Study the drawing (mm; zero at the part's minimum x, y, z) and answer. A direction names the side the tool comes from. Give positions to 0.01 mm unless a question says otherwise; leave off trailing zeros. Write each loop counter-clockwise with the first axis right and the second up, starting at its lowest first coordinate (ties: lowest second). Pieces come first, ordered by that corner, then holes. Notation, with made-up numbers: (11, 36) - (36, 36) arc R23 cw to (36, 52) - close; hole circle Ø7 at (-17, 50.5). An arc over 180 degrees is marked (long way). One line per item, written item: value. Start each with the question number.
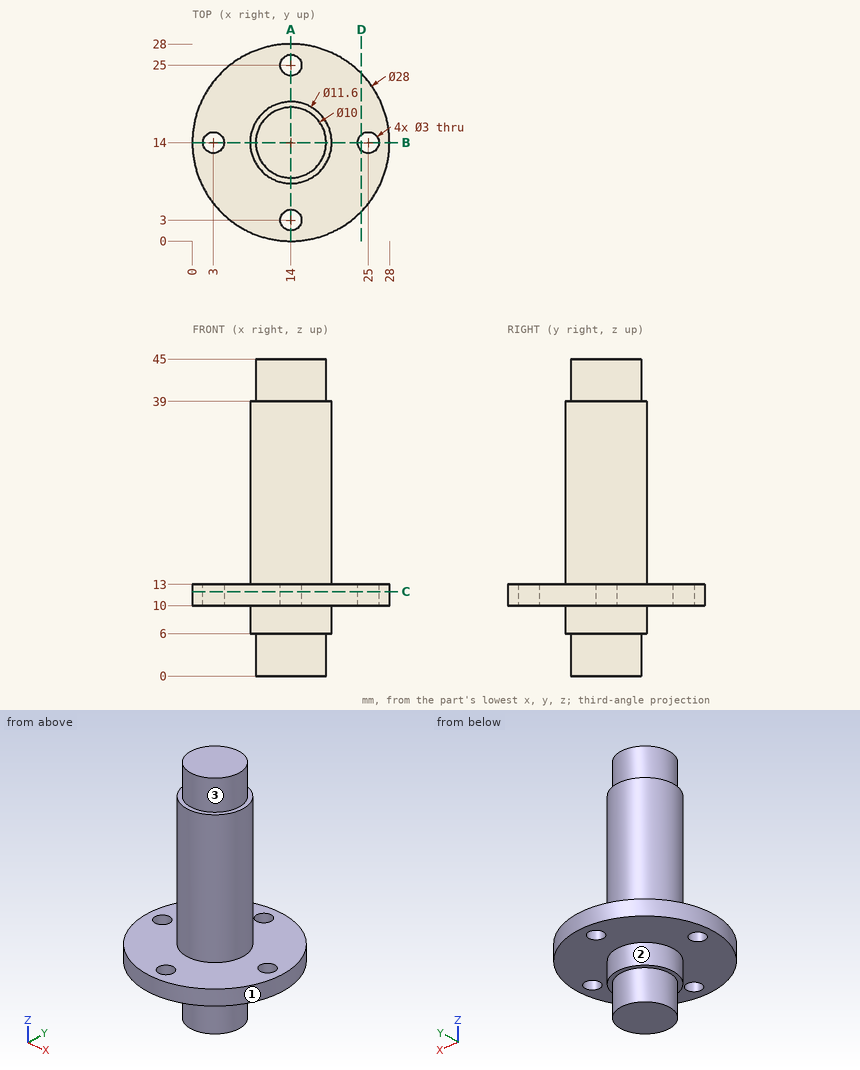
Item 1: For the marked faces 1, 2 and 3, determine the directions among +Z, -Z, +X, -X, +Y, -Y from which every point of the face is accessible in a straight line to the end or side of a thin tool.
Item 2: Each of these flat-tipped pins is pushed along its axis until it touches: pin 1 Ø10 at (y, z) = (23.5, 38) entering from +X; pin 2 Ø10 at (y, z) = (7.5, 7.5) entering from -X; pin 3 Ø5 at (x, y) = (3, 14) entering from +Z; pin 4 Ø13 at (x, y) = (13, 14.5) entering from -Z. Where does it stop, or does it pass through?
Item 3: Straight lines are drawn through the part: line 1 along Y through (x, z) = (14, 11.9); line 2 along Z through (x, y) = (16, 2); line 3 along Y through (x, z) = (3, 11.1). For each, find the intervals that lie inside material, in ascending order.
Item 4: Find section D-D on x = 24. Determine the outline of the cut face in (y, z), plus the area to 3 significant figures.
Item 5: Find section A-A on x = 14. Determine the outline of the cut face in (y, z).
Item 6: Find section C-C on z = 12. Determine the outline of the cut face in (x, y).
Values:
1. face 1: +Z, -Z
1. face 2: -Z
1. face 3: +Z
2. pin 1: x = 17.66
2. pin 2: x = 0.17
2. pin 3: z = 13
2. pin 4: z = 0
3. line 1: 0 to 1.5, 4.5 to 23.5, 26.5 to 28
3. line 2: 10 to 13
3. line 3: 5.34 to 12.5, 15.5 to 22.66
4. outline: (4.2, 10) - (12.88, 10) - (12.88, 13) - (4.2, 13) - close; (15.12, 10) - (23.8, 10) - (23.8, 13) - (15.12, 13) - close
4. area: 52.1 mm^2
5. outline: (0, 10) - (1.5, 10) - (1.5, 13) - (0, 13) - close; (4.5, 10) - (8.2, 10) - (8.2, 6) - (9, 6) - (9, 0) - (19, 0) - (19, 6) - (19.8, 6) - (19.8, 10) - (23.5, 10) - (23.5, 13) - (19.8, 13) - (19.8, 39) - (19, 39) - (19, 45) - (9, 45) - (9, 39) - (8.2, 39) - (8.2, 13) - (4.5, 13) - close; (26.5, 10) - (28, 10) - (28, 13) - (26.5, 13) - close
6. outline: circle Ø28 at (14, 14); hole circle Ø3 at (3, 14); hole circle Ø3 at (14, 3); hole circle Ø3 at (14, 25); hole circle Ø3 at (25, 14)
